Can you work these out from the model? Positions are in its coordinate system, mm. A direction names the side the tool comes from. Coordinates: 2 decimals unless noted, no trailing zeros. Order: outer loops, then holes, each group sorted by start corner. A loop starts at its lowest first (then second) coordinate and runs counter-clockwise, first axis right, second up. Notation, with made-up numbers: (57, 65) - (89, 65) arc R5 ccw to (89, 69) - close; hole circle Ø8 at (54, -2.5). An arc over 180 degrees is marked (long way). Return JSON: item names as keys, results as strings. Group by question number.
1) Imagine slicing it at C-C (z = 3.2). Write out the boundary of the cut face in (x, y), and give its area (3 significant figures).
2) For pin 1 Ø3 at (y, z) = (66.5, 1) entering from -X; pin 2 Ø1.5 at (x, z) = (7, 1.5) entering from -Y; pin 3 Ø3.5 at (x, y) = (-9.9, -9.9) entering from +Z; pin 4 Ø1 at (y, z) = (64, 3.5) entering from +X, each with a flat end and sliding along its axis, tell me the tip position at first contact or that it passes through.
3) If I drill on line 1 along X through (y, z) = (66, 4.45); line 2 along X through (y, z) = (53.5, 3.1); line 3 along Y through (x, z) = (-5.5, 0.55), over which ranges is the centre line in solid material (lowest first)?
4) Imagine slicing it at A-A (y = 92). Write out the boundary of the cut face in (x, z).
5) Which directions (+Z, -Z, +X, -X, +Y, -Y) give clear straight access to the entire face, cutting with the end or side of a thin tool? Please do faces 5 (the face through (0, 33, 0)), 6 (the face through (10, 63, 2)), 7 (the face through (-6.6, 84, 2)).
6) If we mould it in two halves opening along X, with no side actions, what happens to faces 1 (the face through (10.25, -8.34, 2.46)), 2 (the face through (-10, 65, 2)), 3 (the face through (-5, 58.4, 2.5)), 4 (the face through (0, 33, 5))? For each: pulls with the +X half, pulls with the -X half, needs draft (parallel to the pull), parting line crosses it, or undercut.
7) Imagine slicing it at D-D (y = 29.5). Write out the boundary of the cut face in (x, z), and give its area (3 significant figures).
8) Imagine slicing it at B-B (x = 5). Write out the boundary of the cut face in (y, z).
```python
from build123d import *

# Parameters (mm, degrees)
SKETCH_1_R      = 1.6
EXTRUDE_1_DEPTH = 5


with BuildPart() as part:
    # 草图1 → 凸台-拉伸1 (new body)
    with BuildSketch(Plane.XY):
        with BuildLine():
            Line((-10, 110), (-10, 17.88854382))
            ThreePointArc((-10, 17.88854382), (-10.522774425, 15.439054077), (-12, 13.416407865))
            ThreePointArc((-12, 13.416407865), (0, -18), (12, 13.416407865))
            ThreePointArc((12, 13.416407865), (10.522774425, 15.439054077), (10, 17.88854382))
            Line((10, 17.88854382), (10, 110))
            ThreePointArc((10, 110), (9.414213562, 111.414213562), (8, 112))
            Line((8, 112), (-8, 112))
            ThreePointArc((-8, 112), (-9.414213562, 111.414213562), (-10, 110))
        make_face()
        with Locations((-9.899494937, -9.899494937)):
            Circle(SKETCH_1_R, mode=Mode.SUBTRACT)
        with Locations(Location((9.899494937, -9.899494937, 0), (0, 0, 180))):
            Circle(SKETCH_1_R, mode=Mode.SUBTRACT)
        with BuildLine():
            Line((-3.4, 108), (-3.4, 60))
            ThreePointArc((-3.4, 60), (-5, 58.4), (-6.6, 60))
            Line((-6.6, 60), (-6.6, 108))
            ThreePointArc((-6.6, 108), (-5, 109.6), (-3.4, 108))
        make_face(mode=Mode.SUBTRACT)
        with BuildLine():
            Line((3.4, 108), (3.4, 60))
            ThreePointArc((3.4, 60), (5, 58.4), (6.6, 60))
            Line((6.6, 60), (6.6, 108))
            ThreePointArc((6.6, 108), (5, 109.6), (3.4, 108))
        make_face(mode=Mode.SUBTRACT)
    extrude(amount=EXTRUDE_1_DEPTH)


solid = part.part
```
Calculated:
{
 "1": {"outline": "(-12, 13.42) arc R18 ccw (long way) to (12, 13.42) arc R6 cw to (10, 17.89) - (10, 110) arc R2 ccw to (8, 112) - (-8, 112) arc R2 ccw to (-10, 110) - (-10, 17.89) arc R6 cw to start; hole circle Ø3.2 at (-9.9, -9.9); hole (-6.6, 60) arc R1.6 ccw to (-3.4, 60) - (-3.4, 108) arc R1.6 ccw to (-6.6, 108) - close; hole (3.4, 60) arc R1.6 ccw to (6.6, 60) - (6.6, 108) arc R1.6 ccw to (3.4, 108) - close; hole circle Ø3.2 at (9.9, -9.9)", "area": "2,580 mm2"},
 "2": {"pin 1": "x = -10", "pin 2": "y = -16.88", "pin 3": "z = 5", "pin 4": "x = 10"},
 "3": {"line 1": "-10 to -6.6, -3.4 to 3.4, 6.6 to 10", "line 2": "-10 to 10", "line 3": "-17.14 to 58.48, 109.52 to 112"},
 "4": {"outline": "(-10, 0) - (-6.6, 0) - (-6.6, 5) - (-10, 5) - close; (-3.4, 0) - (3.4, 0) - (3.4, 5) - (-3.4, 5) - close; (6.6, 0) - (10, 0) - (10, 5) - (6.6, 5) - close"},
 "5": {"face 5": "-Z, +X, -X, +Y, -Y", "face 6": "+Z, -Z, +X, +Y", "face 7": "+Z, -Z"},
 "6": {"face 1": "undercut", "face 2": "pulls with the -X half", "face 3": "undercut", "face 4": "needs draft"},
 "7": {"outline": "(-10, 0) - (10, 0) - (10, 5) - (-10, 5) - close", "area": "100 mm2"},
 "8": {"outline": "(-17.29, 0) - (58.4, 0) - (58.4, 5) - (-17.29, 5) - close; (109.6, 0) - (112, 0) - (112, 5) - (109.6, 5) - close"}
}
